from build123d import *

# Parameters (mm, degrees)
SKETCH1_W            = 100
SKETCH1_H            = 75
BOSS_EXTRUDE1_DEPTH  = 1.5875
SKETCH2_W            = 20.53
SKETCH2_H            = 3.8
BOSS_EXTRUDE2_DEPTH  = 4.5875
LPATTERN1_COUNT      = 4
LPATTERN1_PITCH      = 24
LPATTERN1_COUNT_DIR2 = 2
LPATTERN1_PITCH_DIR2 = 25


with BuildPart() as part:
    # Sketch1 → Boss-Extrude1 (new body)
    with BuildSketch(Plane(origin=(0, 0, 0), x_dir=(1, 0, 0), z_dir=(0, 1, 0))):
        with Locations((50, 37.5)):
            Rectangle(SKETCH1_W, SKETCH1_H)
    extrude(amount=BOSS_EXTRUDE1_DEPTH)

    # Sketch2 → Boss-Extrude2 (add)
    with BuildSketch(Plane(origin=(0, 0, 0), x_dir=(1, 0, 0), z_dir=(0, 1, 0))):
        with Locations((13.985, 37.4)):
            Rectangle(SKETCH2_W, SKETCH2_H)
    boss_extrude2 = extrude(amount=BOSS_EXTRUDE2_DEPTH)

    # LPattern1: Boss-Extrude2 4 × 2
    with Locations(*[(i * LPATTERN1_PITCH, 0, -j * LPATTERN1_PITCH_DIR2) for i in range(LPATTERN1_COUNT) for j in range(LPATTERN1_COUNT_DIR2) if (i, j) != (0, 0)]):
        add(boss_extrude2)


solid = part.part
Source: CAD feature listing. Evaluate the final solid. Frame: model axes, mm. A direction names the side the tool comes from. Round coordinates to 2 decimals unless told otherwise and drop trailing zeros. Loops run counter-clockwise (first coordinate to the right, second up) from the corner with the lowest first, then second, coordinate; pieces in that order, holes last.
Q1. Section B-B, the plane x = 17.5. Return loops of the section in (y, z), plus the area to 3 significant figures.
Q2. First-contact query: P1, Ø1.5, axis at x = 61, z = -52, coming from the +Y side; P2, Ø1.5, axis at y = 3.5, z = -63, coming from the -X side; P3, Ø1.5, axis at x = 15.5, y = 3, coming from the +Z side. Flat tips, straight axial feed; report the tip coordinate or a pass-through.
Q3. Section A-A, the plane y = 3.6. State how many separate pieces and enclosed holes the cut face has, plus the area to 3 significant figures.
Q4. Section C-C, the plane z = -47. Return loops of the section in (x, y).
Q5. Mould query, pull axis X, two halves, no side actions, for faces 1 (the face through (75.72, 3, -62)), 2 (the face through (86, 3, -64.3)), 3 (the face through (51.72, 3, -37)), 4 (the face through (96.25, 3, -62)). Classes: pulls with the +X half, pulls with the -X half, needs draft (parallel to the pull), parting line crosses it, or undercut.
Q6. Ray query, line 1 (Z direction, x = 8, y = 2.8); line 2 (X direction, y = 4.2, z = -61); line 3 (Y direction, x = 26.5, z = -20). Return the intervals inside material, ascending.
Q7. Access query for faces 5 (the face through (86, 3, -35.5)), 6 (the face through (27.72, 3, -62)), 7 (the face through (14, 3, -39.3)). Directions: +Z, -Z, +X, -X, +Y, -Y. A direction counts if a zero-diameter tool reaches every point of the face in a straight line with its end or side. Return the directions, or none.
Solutions:
1. outline: (0, -75) - (1.59, -75) - (1.59, -64.3) - (4.59, -64.3) - (4.59, -60.5) - (1.59, -60.5) - (1.59, -39.3) - (4.59, -39.3) - (4.59, -35.5) - (1.59, -35.5) - (1.59, 0) - (0, 0) - close
1. area: 142 mm2
2. P1: stops at y = 1.59
2. P2: stops at x = 3.72
2. P3: stops at z = -35.5
3. separate pieces: 8
3. enclosed holes: 0
3. area: 624 mm2
4. outline: (0, 0) - (100, 0) - (100, 1.59) - (0, 1.59) - close
5. face 1: undercut
5. face 2: needs draft
5. face 3: undercut
5. face 4: pulls with the +X half
6. line 1: z = -64.3 to -60.5, -39.3 to -35.5
6. line 2: x = 3.72 to 24.25, 27.72 to 48.25, 51.72 to 72.25, 75.72 to 96.25
6. line 3: y = 0 to 1.59
7. face 5: +Z, +X, -X, +Y
7. face 6: +Z, -Z, +Y
7. face 7: +X, -X, +Y
